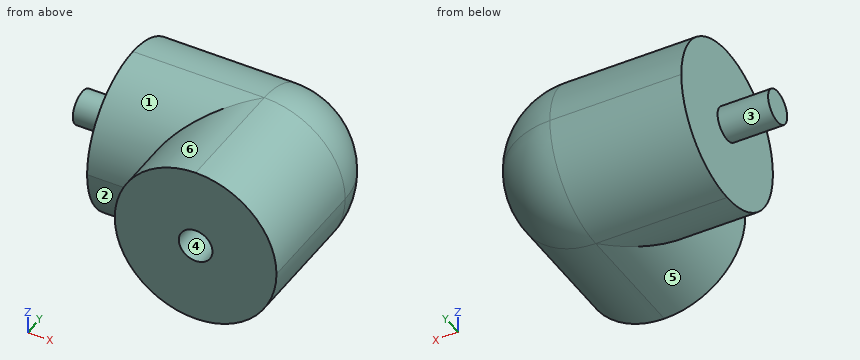
```python
from build123d import *

# Parameters (mm, degrees)
SKETCH1_W           = 48
SKETCH1_H           = 48
BOSS_EXTRUDE1_DEPTH = 30
SKETCH3_W           = 48
SKETCH3_H           = 48
BOSS_EXTRUDE2_DEPTH = 15
FILLET1_R           = 24
SKETCH4_R           = 5
CUT_EXTRUDE1_DEPTH  = 15
SKETCH5_R           = 5
BOSS_EXTRUDE3_DEPTH = 15


with BuildPart() as part:
    # Sketch1 → Boss-Extrude1 (new, symmetric)
    with BuildSketch(Plane(origin=(0, 0, 0), x_dir=(1, 0, 0), z_dir=(0, 1, 0))):
        with Locations((24, 24)):
            Rectangle(SKETCH1_W, SKETCH1_H)
    extrude(amount=BOSS_EXTRUDE1_DEPTH, both=True)

    # Sketch3 → Boss-Extrude2 (add)
    with BuildSketch(Plane.ZY):
        with Locations((-24, 6)):
            Rectangle(SKETCH3_W, SKETCH3_H)
    extrude(amount=BOSS_EXTRUDE2_DEPTH)

    # Fillet1
    fillet1_edges = [part.edges().sort_by_distance(p)[0] for p in [
        (48, 30, -24),
        (0, -24, 0),
        (0, -24, -48),
        (-7.5, -18, -48),
        (16.5, 30, -48),
        (-7.5, -18, 0),
        (48, 0, -48),
        (48, 0, 0),
        (16.5, 30, 0),
    ]]
    fillet(fillet1_edges, radius=FILLET1_R - 0.0001)  # a hair under: the kernel refuses the full size

    # Sketch4 → Cut-Extrude1 (cut)
    with BuildSketch(Plane(origin=(0, -30, 0), x_dir=(-1, 0, 0), z_dir=(0, -1, 0))):
        with Locations(Location((-24, 24, 0), (0, 0, 90))):
            Circle(SKETCH4_R)
    extrude(amount=-CUT_EXTRUDE1_DEPTH, mode=Mode.SUBTRACT)

    # Sketch5 → Boss-Extrude3 (add)
    with BuildSketch(Plane.ZY.offset(15)):
        with Locations((-24, 6)):
            Circle(SKETCH5_R)
    extrude(amount=BOSS_EXTRUDE3_DEPTH)


solid = part.part
```
For this review, take the finished solid that the model builds, in its own axes (mm). Face numbers are marked on the shaded views. A direction names the side the tool comes from. Coordinates: 2 decimals unless noted, no trailing zeros. Loops run counter-clockwise (first coordinate to the right, second up) from the corner with the lowest first, then second, coordinate; pieces in that order, holes last. Notation, with made-up numbers: (76, -32.75) - (125, -32.75) arc R16 ccw to (125, -14.75) - close; hole circle Ø5 at (-38.5, 55.25). An arc over 180 degrees is marked (long way). Use one line per item in the form item = value. Start each with the question number.
1) Take a section at B-B (z = -30.5). State the section outline as (x, y) points, plus the area to 3 significant figures.
2) For pin 1 (2 mm diameter, centred on y = 0.5, z = -32.5, fed in from -X); pin 2 (1.5 mm diameter, centred on x = 29, y = 19, fed in from -Z); pin 3 (5 mm diameter, centred on y = -5, z = -32, fed in from +X), all flat-tipped, find the tip position at first contact; note any pin that passes through.
3) To check wall thickness, follow probe 1 along X at (y, z) = (-25.75, -24); probe 2 along X at (y, z) = (-24.5, -21); probe 3 along X at (y, z) = (-3, -24). State the ranges of each line that lie inside material, in increasing order. Write a range as from..to.
4) Draft analysis for pull direction Z (two halves, no side actions). For the marked faces 4, 5 and 6, state which applies: released by +Z, released by -Z, zero draft, split by the parting line, or undercut.
5) Take a section at D-D (z = -8). State the section outline as (x, y) points.
6) For the marked faces 1, 2 and 3, list the 3-axis set-ups (+Z, -Z, +X, -X, +Y, -Y) from which the entire face can be reached by the end or side of a thin tool; tool diameter is ignored.
From the geometry:
q1.outline = (-15, -17.1) - (0.9, -17.1) - (0.9, -30) - (47.1, -30) - (47.1, 6) arc R23.1 ccw to (24, 29.1) - (-15, 29.1) - close
q1.area = 3,350 mm2
q2.pin_1 = -15
q2.pin_2 = -44.06
q2.pin_3 = 47.36
q3.probe_1 = 0..19, 29..48
q3.probe_2 = 0.19..20, 28..47.81
q3.probe_3 = -15..48
q4.face_4 = undercut
q4.face_5 = released by -Z
q4.face_6 = released by +Z
q5.outline = (-15, -11.89) - (6.11, -11.89) - (6.11, -30) - (41.89, -30) - (41.89, 6) arc R17.89 ccw to (24, 23.89) - (-15, 23.89) - close
q6.face_1 = +Z, -X, -Y
q6.face_2 = -Z, -X, -Y
q6.face_3 = -X
